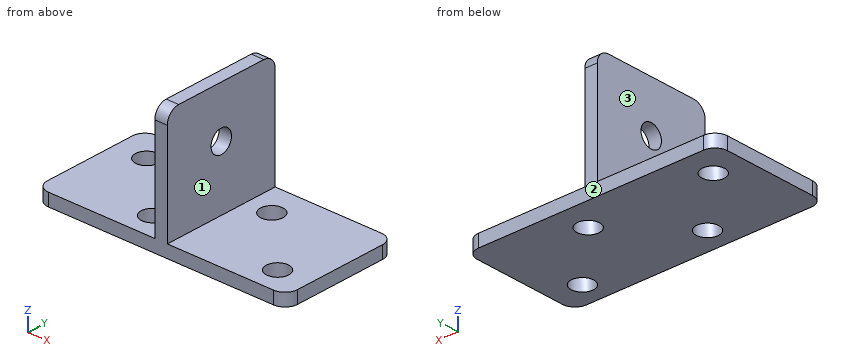
from build123d import *

# Parameters (mm, degrees)
F1_DEPTH = 47.5
F2_R     = 9
F3_DEPTH = 25
F4_R     = 9
F5_DEPTH = 25
F6_R     = 10


with BuildPart() as f1:
    # F0 (on Front) → F1 (new body, symmetric)
    with BuildSketch(Plane.XZ):
        Polygon((-100, 0), (0, 0), (100, 0), (100, 10), (5, 10), (5, 100), (0, 100), (-5, 100), (-5, 10), (-100, 10), align=None)
    extrude(amount=F1_DEPTH, both=True)

    # F2 (on face) → F3 (cut)
    with BuildSketch(Plane.XY.offset(10)):
        with Locations((75, -27.5)):
            Circle(F2_R)
        with Locations((25, 22.5)):
            Circle(F2_R)
        with Locations((-25, -27.5)):
            Circle(F2_R)
        with Locations((-75, 22.5)):
            Circle(F2_R)
    extrude(amount=-F3_DEPTH, mode=Mode.SUBTRACT)

    # F4 (on face) → F5 (cut)
    with BuildSketch(Plane(origin=(-5, 0, 0), x_dir=(0, -1, 0), z_dir=(-1, 0, 0))):
        with Locations((0, 60)):
            Circle(F4_R)
    extrude(amount=-F5_DEPTH, mode=Mode.SUBTRACT)

    # F6
    f6_edges = [f1.edges().sort_by_distance(p)[0] for p in [
        (0, -47.5, 100),
        (0, 47.5, 100),
        (-100, 47.5, 5),
        (-100, -47.5, 5),
        (100, 47.5, 5),
        (100, -47.5, 5),
    ]]
    fillet(f6_edges, radius=F6_R)


solid = f1.part
Geometry: final body of the model. Coordinates: model frame, mm. Face numbers are marked on the shaded views. A direction names the side the tool comes from. Round coordinates to 2 decimals unless told otherwise and drop trailing zeros. Loops run counter-clockwise (first coordinate to the right, second up) from the corner with the lowest first, then second, coordinate; pieces in that order, holes last. Notation, with made-up numbers: (-21, 25) -> (21, 25) arc R33 ccw to (21, 54) -> close; hole circle Ø5 at (68, -10.75). An arc over 180 degrees is marked (long way). One line per question, with ' | ' between items. Start each with the question number.
1. Section C-C on z = 54.5. Output: boundary loops of the cut face in (x, y), and give its area (3 significant figures).
2. Section A-A on x = 75. Output: boundary loops of the cut face in (y, z).
3. Set-up query: the marked faces 1, 2 and 3. Return all of +Z, -Z, +X, -X, +Y, -Y with unobstructed straight access to the full face (end or side cutting, diameter ignored); none if empty.
4. Contact query for flat-ended pins moving along their axis: pin 1 (16 mm diameter, centred on x = 75, y = -27.5, fed in from -Z); pin 2 (2 mm diameter, centred on x = 61.5, y = 16, fed in from +Z); pin 3 (12 mm diameter, centred on y = -19.5, z = 61.5, fed in from -X). Output: stop coordinate, or through.
5. Line query: line 1 along X through (y, z) = (22, 4); line 2 along Y through (x, z) = (-75, 7.5); line 3 along Z through (x, y) = (-2, 0). Output: solid intervals per line, ascending. Write a range as [from, to].
6. Section B-B on y = -27.5. Output: boundary loops of the cut face in (x, z), and give its area (3 significant figures).
7. Section D-D on x = 12. Output: boundary loops of the cut face in (y, z).
Returned:
1) outline: (-5, -47.5) -> (5, -47.5) -> (5, -7.12) -> (-5, -7.12) -> close; (-5, 7.12) -> (5, 7.12) -> (5, 47.5) -> (-5, 47.5) -> close | area: 808 mm2
2) outline: (-47.5, 0) -> (-36.5, 0) -> (-36.5, 10) -> (-47.5, 10) -> close; (-18.5, 0) -> (47.5, 0) -> (47.5, 10) -> (-18.5, 10) -> close
3) face 1: +Z, +X, +Y, -Y | face 2: +Z, -Z, +X, -X, +Y | face 3: +Z, -X, +Y, -Y
4) pin 1: passes through | pin 2: stops at z = 10 | pin 3: stops at x = -5
5) line 1: x = [-100, -83.99], [-66.01, 16.01], [33.99, 100] | line 2: y = [-47.5, 13.5], [31.5, 47.5] | line 3: z = [0, 51], [69, 100]
6) outline: (-100, 0) -> (-34, 0) -> (-34, 10) -> (-100, 10) -> close; (-16, 0) -> (66, 0) -> (66, 10) -> (5, 10) -> (5, 100) -> (-5, 100) -> (-5, 10) -> (-16, 10) -> close; (84, 0) -> (100, 0) -> (100, 10) -> (84, 10) -> close | area: 2,540 mm2
7) outline: (-47.5, 0) -> (47.5, 0) -> (47.5, 10) -> (-47.5, 10) -> close
